Part print with two shaded views. Sizes in mm from the minimum x, y, z corner. Give positions to 0.01 mm unless a question says otherwise; leave off trailing zeros. Loops run counter-clockwise (first coordinate to the right, second up) from the corner with the lowest first, then second, coordinate; pieces in that order, holes last. Notation, with made-up numbers: M 52,4 L 102,4 A13 cw 102,16 Z; hole C 87.5,-4.75 d6. An arc over 180 degrees is marked long. Answer in a Markdown table with one row per item.
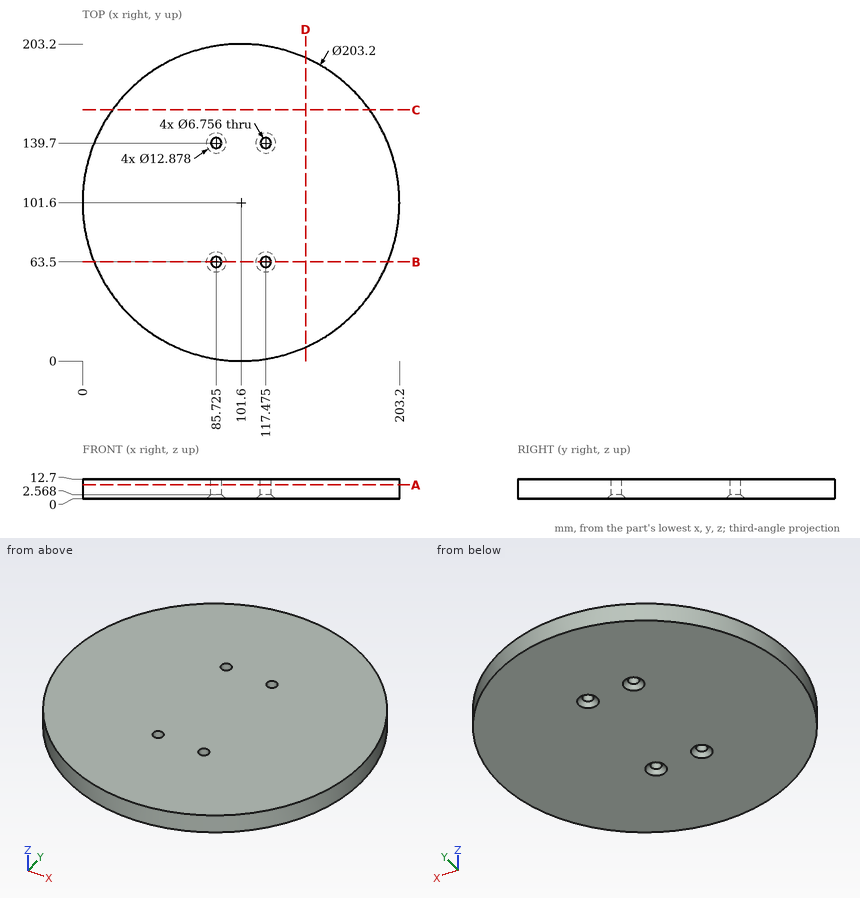
Q1. Saw through at C-C (y = 161). Give the cut face in (x, z).
Reported:
| item | result |
|---|---|
| outline | M 19.17,0 L 184.03,0 L 184.03,12.7 L 19.17,12.7 Z |
Q2. Saw through at D-D (x = 143). Give the cut face in (y, z).
Reported:
| item | result |
|---|---|
| outline | M 8.82,0 L 194.38,0 L 194.38,12.7 L 8.82,12.7 Z |
Q3. Saw through at A-A (z = 9). Give the cut face in (x, y) (1 decimal).
Reported:
| item | result |
|---|---|
| outline | C 101.6,101.6 d203.2; hole C 85.7,63.5 d6.8; hole C 85.7,139.7 d6.8; hole C 117.5,63.5 d6.8; hole C 117.5,139.7 d6.8 |
Q4. Probe probe 1 along X at (y, z) = (63.5, 8) (1 decimal); probe 2 along Y at (x, z) = (120, 11.25) (1 decimal); probe 3 along Y at (x, z) = (103, 8.75). List the from-to ranges inside material, lowest first.
Reported:
| item | result |
|---|---|
| probe 1 | 7.4 to 82.3, 89.1 to 114.1, 120.9 to 195.8 |
| probe 2 | 1.7 to 61.3, 65.7 to 137.5, 141.9 to 201.5 |
| probe 3 | 0.01 to 203.19 |
Q5. Saw through at B-B (y = 63.5). Give the cut face in (x, z) (1 decimal).
Reported:
| item | result |
|---|---|
| outline | M 7.4,0 L 79.3,0 L 82.3,2.6 L 82.3,12.7 L 7.4,12.7 Z; M 89.1,2.6 L 92.2,0 L 111,0 L 114.1,2.6 L 114.1,12.7 L 89.1,12.7 Z; M 120.9,2.6 L 123.9,0 L 195.8,0 L 195.8,12.7 L 120.9,12.7 Z |
Q6. Drop flat-ended pins along their axis: pin 1 (2 mm diameter, centred on y = 163.5, z = 7.5, fed in from -X) (1 decimal); pin 2 (6 mm diameter, centred on x = 85.725, y = 63.5, fed in from -Z); pin 3 (6 mm diameter, centred on y = 26, z = 1.5, fed in from +X) (1 decimal); pin 4 (6 mm diameter, centred on y = 51.5, z = 1.5, fed in from -X). Give the stop position or say it passes through.
Reported:
| item | result |
|---|---|
| pin 1 | x = 20.3 |
| pin 2 | through |
| pin 3 | x = 172.7 |
| pin 4 | x = 11.58 |
